Geometry check sheet. Reference: the model listing, model coordinates, mm. A direction names the side the tool comes from. Give positions to 0.01 mm unless a question says otherwise; leave off trailing zeros. Write each loop counter-clockwise with the first axis right and the second up, starting at its lowest first coordinate (ties: lowest second). Pieces come first, ordered by that corner, then holes. Notation, with made-up numbers: (31, 42) - (48, 42) arc R21 cw to (48, 55) - close; hole circle Ø8 at (-9.5, 57.25). An arc over 180 degrees is marked (long way). Use a Markdown table: item, result.
```python
from build123d import *

# Parameters (mm, degrees)
SKETCH_1_W          = 3
SKETCH_1_H          = 24
EXTRUDE_1_DEPTH     = 16
SKETCH_2_R          = 1.5
CUT_EXTRUDE_1_DEPTH = 16
CHAMFER_1_SIZE      = 1
SKETCH_3_W          = 16
SKETCH_3_H          = 3
EXTRUDE_2_DEPTH     = 10
EXTRUDE_3_DEPTH     = 3
CHAMFER_2_SIZE      = 1
SKETCH_5_R          = 1.5
CUT_EXTRUDE_2_DEPTH = 10
CHAMFER_3_SIZE      = 7


with BuildPart() as part:
    # 草图1 → 凸台-拉伸1 (new body)
    with BuildSketch(Plane.XY):
        with Locations((-1.5, 12)):
            Rectangle(SKETCH_1_W, SKETCH_1_H)
    extrude(amount=EXTRUDE_1_DEPTH)

    # 草图2 → 切除-拉伸1 (cut)
    with BuildSketch(Plane.ZY.offset(3)):
        with Locations((4, 4)):
            Circle(SKETCH_2_R)
        with Locations((12, 4)):
            Circle(SKETCH_2_R)
        with Locations((4, 20)):
            Circle(SKETCH_2_R)
        with Locations((12, 20)):
            Circle(SKETCH_2_R)
    extrude(amount=-CUT_EXTRUDE_1_DEPTH, mode=Mode.SUBTRACT)

    # 倒角1
    chamfer_1_edges = [part.edges().sort_by_distance(p)[0] for p in [
        (-1.5, 24, 0),
        (-1.5, 24, 16),
    ]]
    chamfer(chamfer_1_edges, length=CHAMFER_1_SIZE)

    # 草图3 → 凸台-拉伸2 (add)
    with BuildSketch(Plane(origin=(0, 0, 0), x_dir=(0, 0, -1), z_dir=(1, 0, 0))):
        with Locations((-8, -1.5)):
            Rectangle(SKETCH_3_W, SKETCH_3_H)
    extrude(amount=-EXTRUDE_2_DEPTH)

    # 草图4 → 凸台-拉伸3 (add)
    with BuildSketch(Plane(origin=(0, 0, 0), x_dir=(1, 0, 0), z_dir=(0, 1, 0))):
        Polygon((-10, 11), (-46, 11), (-46, -3), (-10, -3), (-10, 0), align=None)
        Polygon((-10, -16), (-10, -13), (-46, -13), (-46, -27), (-10, -27), align=None)
    extrude(amount=-EXTRUDE_3_DEPTH)

    # 倒角2
    chamfer_2_edges = [part.edges().sort_by_distance(p)[0] for p in [
        (-46, -1.5, 3),
        (-46, -1.5, -11),
        (-10, -1.5, -11),
        (-46, -1.5, 27),
        (-10, -1.5, 27),
        (-46, -1.5, 13),
    ]]
    chamfer(chamfer_2_edges, length=CHAMFER_2_SIZE)

    # 草图5 → 切除-拉伸2 (cut)
    with BuildSketch(Plane(origin=(0, 0, 0), x_dir=(1, 0, 0), z_dir=(0, 1, 0))):
        with Locations((-40, 8)):
            Circle(SKETCH_5_R)
        with Locations((-32, 8)):
            Circle(SKETCH_5_R)
        with Locations((-24, 8)):
            Circle(SKETCH_5_R)
        with Locations((-16, 8)):
            Circle(SKETCH_5_R)
        with Locations((-40, 0)):
            Circle(SKETCH_5_R)
        with Locations((-32, 0)):
            Circle(SKETCH_5_R)
        with Locations((-24, 0)):
            Circle(SKETCH_5_R)
        with Locations((-16, 0)):
            Circle(SKETCH_5_R)
        with Locations((-40, -16)):
            Circle(SKETCH_5_R)
        with Locations((-40, -24)):
            Circle(SKETCH_5_R)
        with Locations((-32, -16)):
            Circle(SKETCH_5_R)
        with Locations((-32, -24)):
            Circle(SKETCH_5_R)
        with Locations((-24, -16)):
            Circle(SKETCH_5_R)
        with Locations((-24, -24)):
            Circle(SKETCH_5_R)
        with Locations((-16, -16)):
            Circle(SKETCH_5_R)
        with Locations((-16, -24)):
            Circle(SKETCH_5_R)
    extrude(amount=-CUT_EXTRUDE_2_DEPTH, mode=Mode.SUBTRACT)

    # 倒角3
    chamfer_3_edges = [part.edges().sort_by_distance(p)[0] for p in [
        (-10, -1.5, 16),
        (-10, -1.5, 0),
    ]]
    chamfer(chamfer_3_edges, length=CHAMFER_3_SIZE)


solid = part.part
```
1) Mould release check, pull along Z, two halves, no side actions. Record for faces 1 (the flat face through (-28, -3, -1)), 2 (the cylindrical face through (-33.2, -1.5, 0.9)), 3 (the flat face through (-28, -1, 27)): pulls with the +Z half, pulls with the -Z half, needs draft (parallel to the pull), parting line crosses it, or undercut.
Working result:
| item | result |
|---|---|
| face 1 | needs draft |
| face 2 | undercut |
| face 3 | pulls with the +Z half |
2) Set-up check for faces 4 (the flat face through (-28, -1, 3)), 5 (the flat face through (-3, 12, 8)), 6 (the cylindrical face through (-17.5, -1.48, -8.07)): record each of +Z, -Z, +X, -X, +Y, -Y from which the full face is reachable in a straight line by a thin tool's end or side.
Working result:
| item | result |
|---|---|
| face 4 | -X, +Y, -Y |
| face 5 | +Z, -Z, -X, +Y |
| face 6 | +Y, -Y |
3) Section check C-C on y = 20. Record the boundary of the cut face in (x, z).
Working result:
| item | result |
|---|---|
| outline | (-3, 0) - (0, 0) - (0, 2.5) - (-3, 2.5) - close; (-3, 5.5) - (0, 5.5) - (0, 10.5) - (-3, 10.5) - close; (-3, 13.5) - (0, 13.5) - (0, 16) - (-3, 16) - close |
4) Depth check by flat-ended pin: P1, Ø2.5, axis at y = -1.5, z = 25, coming from the +X side; P2, Ø1.5, axis at y = -1, z = 8.5, coming from the -X side; P3, Ø4, axis at x = -40, z = 16, coming from the +Y side. Enter the tip coordinate at first touch or a pass-through.
Working result:
| item | result |
|---|---|
| P1 | stops at x = -10 |
| P2 | stops at x = -10 |
| P3 | stops at y = 0 |
5) Section check B-B on z = -8. Record the boundary of the cut face in (x, y).
Working result:
| item | result |
|---|---|
| outline | (-46, -3) - (-41.5, -3) - (-41.5, 0) - (-46, 0) - close; (-38.5, -3) - (-33.5, -3) - (-33.5, 0) - (-38.5, 0) - close; (-30.5, -3) - (-25.5, -3) - (-25.5, 0) - (-30.5, 0) - close; (-22.5, -3) - (-17.5, -3) - (-17.5, 0) - (-22.5, 0) - close; (-14.5, -3) - (-10, -3) - (-10, 0) - (-14.5, 0) - close |
6) Section check D-D on z = 7.5. Record the boundary of the cut face in (x, y).
Working result:
| item | result |
|---|---|
| outline | (-10, -3) - (0, -3) - (0, 24) - (-3, 24) - (-3, 0) - (-10, 0) - close |
7) Section check A-A on x = -32. Record the boundary of the cut face in (y, z).
Working result:
| item | result |
|---|---|
| outline | (-3, -11) - (0, -11) - (0, -9.5) - (-3, -9.5) - close; (-3, -6.5) - (0, -6.5) - (0, -1.5) - (-3, -1.5) - close; (-3, 1.5) - (0, 1.5) - (0, 3) - (-3, 3) - close; (-3, 13) - (0, 13) - (0, 14.5) - (-3, 14.5) - close; (-3, 17.5) - (0, 17.5) - (0, 22.5) - (-3, 22.5) - close; (-3, 25.5) - (0, 25.5) - (0, 27) - (-3, 27) - close |
8) Material ranges on L1, parallel to X at y = -0.85, z = -8; L2, parallel to Y at x = -1.6, z = 12; L3, parallel to Z at x = -16, y = -0.75, recorded low to high. Write a range as from..to.
Working result:
| item | result |
|---|---|
| L1 | x = -46..-41.5, -38.5..-33.5, -30.5..-25.5, -22.5..-17.5, -14.5..-10 |
| L2 | y = -3..2.5, 5.5..18.5, 21.5..24 |
| L3 | z = -11..-9.5, -6.5..-1.5, 1.5..3, 13..14.5, 17.5..22.5, 25.5..27 |
